from build123d import *

# Parameters (mm, degrees)
SKETCH1_R           = 7.5
SKETCH1_R_2         = 20
BOSS_EXTRUDE3_DEPTH = 15
SKETCH1_9_R         = 20
SKETCH1_9_R_2       = 10
BOSS_EXTRUDE4_DEPTH = 35


with BuildPart() as part:
    # Sketch1 → Boss-Extrude3 (new body)
    with BuildSketch(Plane.XY):
        with BuildLine():
            Line((-11.361079264, -3.667783279), (-1.853421221, 32.520673976))
            ThreePointArc((-1.853421221, 32.520673976), (3.493809463, 40.587118039), (12.654236823, 43.709131232))
            Line((12.654236823, 43.709131232), (102.654236823, 43.709131232))
            ThreePointArc((102.654236823, 43.709131232), (117.619577951, 27.690031183), (100.620746174, 13.847606553))
            ThreePointArc((100.620746174, 13.847606553), (67.179976661, 6.607096754), (46.224814518, -20.440846371))
            ThreePointArc((46.224814518, -20.440846371), (9.264757731, -40.093935282), (-11.361079264, -3.667783279))
        make_face()
        with Locations((12.654236823, 28.709131232)):
            Circle(SKETCH1_R, mode=Mode.SUBTRACT)
        with Locations((17.654236823, -11.290868768)):
            Circle(SKETCH1_R_2, mode=Mode.SUBTRACT)
        with BuildLine():
            Line((62.654236823, 34.709131232), (102.654236823, 34.709131232))
            ThreePointArc((102.654236823, 34.709131232), (108.654236823, 28.709131232), (102.654236823, 22.709131232))
            Line((102.654236823, 22.709131232), (62.654236823, 22.709131232))
            ThreePointArc((62.654236823, 22.709131232), (56.654236823, 28.709131232), (62.654236823, 34.709131232))
        make_face(mode=Mode.SUBTRACT)
    extrude(amount=BOSS_EXTRUDE3_DEPTH)

    # Sketch1<9> → Boss-Extrude4 (add)
    with BuildSketch(Plane.XY):
        with Locations((17.654236823, -11.290868768)):
            Circle(SKETCH1_9_R)
        with Locations((17.654236823, -11.290868768)):
            Circle(SKETCH1_9_R_2, mode=Mode.SUBTRACT)
    extrude(amount=BOSS_EXTRUDE4_DEPTH)


solid = part.part
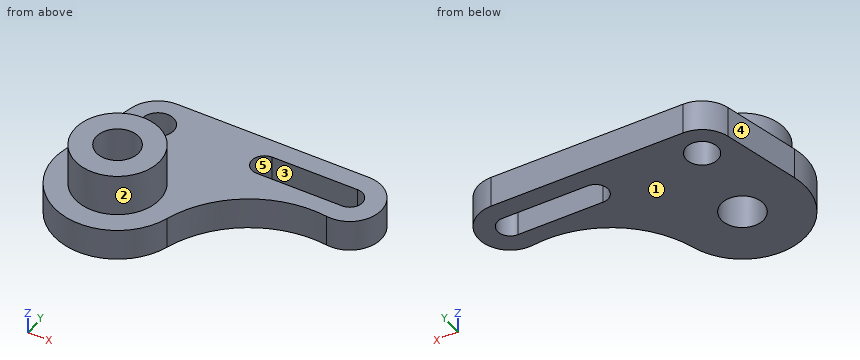
Verification items for the finished model (mm, model axes). Face numbers are marked on the shaded views. A direction names the side the tool comes from. Coordinates: 2 decimals unless noted, no trailing zeros. Order: outer loops, then holes, each group sorted by start corner. A loop starts at its lowest first (then second) coordinate and runs counter-clockwise, first axis right, second up. Notation, with made-up numbers: M -37,70 L -28,70 A25 ccw -28,93 Z; hole C -5,-17.75 d9. An arc over 180 degrees is marked long. Return JSON: item names as keys, results as strings.
1) Cross-section at B-B, the plane y = 25. Record the boundary of the cut face in (x, z), and give its area (3 significant figures).
Answer list:
{"outline": "M -3.83,0 L 6.14,0 L 6.14,15 L -3.83,15 Z; M 19.17,0 L 57.94,0 L 57.94,15 L 19.17,15 Z; M 107.37,0 L 117.19,0 L 117.19,15 L 107.37,15 Z", "area": "878 mm2"}
2) Gauge pin test, flat ends, axial feed: pin 1 (7.5 mm diameter, centred on x = 74.5, z = 6.5, fed in from -Y); pin 2 (6 mm diameter, centred on x = 38, y = 8, fed in from +Z); pin 3 (3 mm diameter, centred on y = 21.5, z = 15.5, fed in from -X). Record the tip position at first contact, or that the pin passes through.
Answer list:
{"pin 1": "y = 8.66", "pin 2": "z = 15", "pin 3": "x = -5.12"}
3) Access from +Z, -Z, +X, -X, +Y, -Y to the whole of each face (thin tool, end or side, straight path). Record for the marked faces 4 and 5.
Answer list:
{"face 4": "+Z, -Z, -X, +Y", "face 5": "+Z, -Z"}
4) Release check for a two-part mould opening along X. For the marked faces 1, 2 and 3 record: +X half, -X half, draft (parallel to the pull), parting line (faces both ways), or undercut.
Answer list:
{"face 1": "draft", "face 2": "parting line", "face 3": "undercut"}
5) Thickness scan on L1, parallel to X at y = 26, z = 9.5; L2, parallel to Z at x = 39.5, y = 16; L3, parallel to X at y = -5, z = 24. Record the ranges inside material, lowest first. Write a range as [from, to].
Answer list:
{"L1": "[-3.57, 5.66], [19.65, 57.3], [108.01, 117.41]", "L2": "[0, 15]", "L3": "[-1.33, 9.88], [25.43, 36.64]"}
6) Cross-section at C-C, the plane z = 6. Record the boundary of the cut face in (x, y), and give its area (3 significant figures).
Answer list:
{"outline": "M -11.36,-3.67 A30 ccw 46.22,-20.44 A50 cw 100.62,13.85 A15 ccw long 102.65,43.71 L 12.65,43.71 A15 ccw -1.85,32.52 Z; hole C 12.65,28.71 d15; hole C 17.65,-11.29 d20; hole M 62.65,22.71 L 102.65,22.71 A6 ccw 102.65,34.71 L 62.65,34.71 A6 ccw Z", "area": "5,630 mm2"}
7) Cross-section at A-A, the plane x = 79.5. Record the boundary of the cut face in (y, z), and give its area (3 significant figures).
Answer list:
{"outline": "M 12.21,0 L 22.71,0 L 22.71,15 L 12.21,15 Z; M 34.71,0 L 43.71,0 L 43.71,15 L 34.71,15 Z", "area": "293 mm2"}
8) Cross-section at D-D, the plane x = 35. Record the boundary of the cut face in (y, z), and give its area (3 significant figures).
Answer list:
{"outline": "M -35.77,0 L 43.71,0 L 43.71,15 L -1.33,15 L -1.33,35 L -21.25,35 L -21.25,15 L -35.77,15 Z", "area": "1,590 mm2"}
